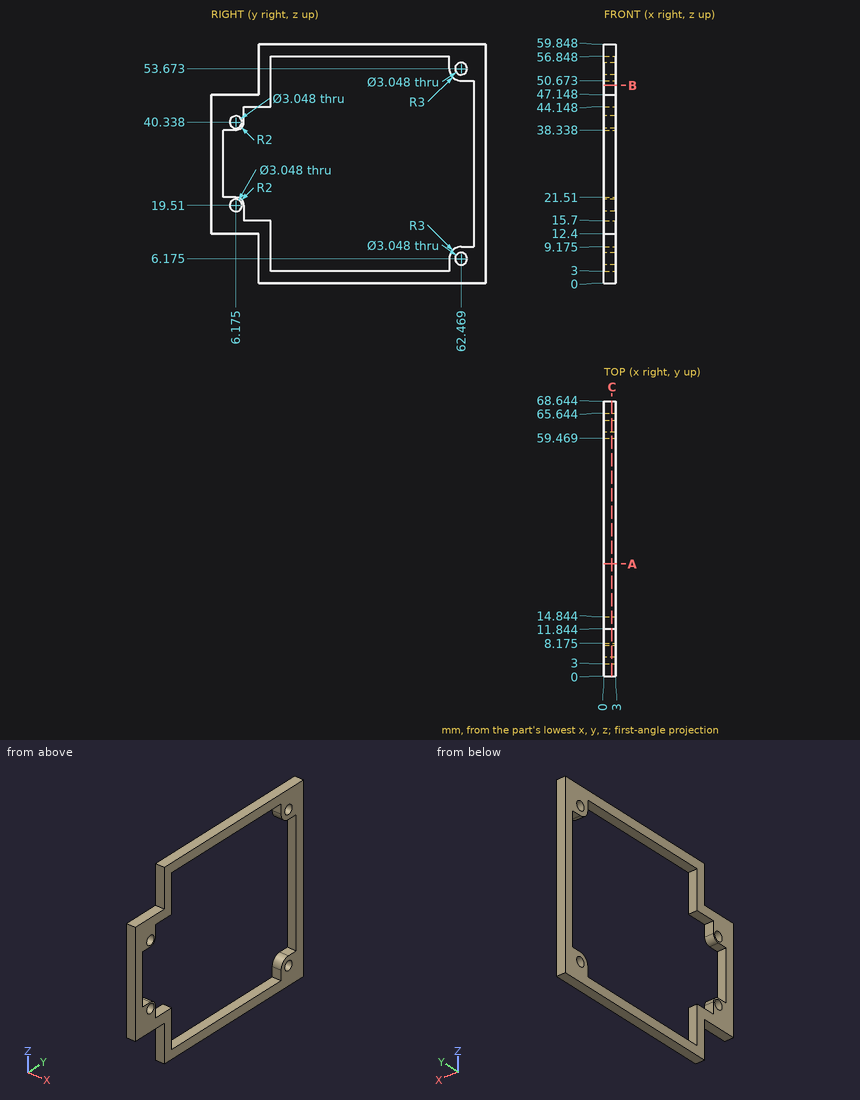
Geometry check sheet. Reference: drawing and pictorial views, mm from the part's lowest x, y, z. Round coordinates to 2 decimals unless told otherwise and drop trailing zeros. Loops run counter-clockwise (first coordinate to the right, second up) from the corner with the lowest first, then second, coordinate; pieces in that order, holes last. Notation, with made-up numbers: (87, 12.25) - (129, 12.25) arc R21 cw to (129, 39.25) - close; hole circle Ø10 at (-31.75, 21). An arc over 180 degrees is marked (long way). Write item = value, one per line. Start each with the question number.
Q1. Section check B-B (z = 49.5). Record the boundary of the cut face in (x, y).
Q2. Depth check by flat-ended pin: P1, Ø0.9, axis at x = 1, z = 55, coming from the -Y side; P2, Ø1.5, axis at x = 1, y = 3.5, coming from the +Z side; P3, Ø2.5, axis at y = 6.175, z = 40.338, coming from the -X side. Enter the tip coordinate at first touch or a pass-through.
Q3. Thickness scan on L1, parallel to Y at x = 0.9, z = 6 (1 decimal); L2, parallel to Z at x = 2.5, y = 56; L3, parallel to Y at x = 1.35, z = 17.5 (1 decimal). Record the ranges inside material, lowest first.
Q4. Section check C-C (x = 2). Count the separate pieces of the cut face and the enclosed holes in it, plus the area to 3 significant figures.
Q5. Section check A-A (y = 28). Record the boundary of the cut face in (x, z).
Derived:
q1.outline = (0, 11.84) - (3, 11.84) - (3, 14.84) - (0, 14.84) - close; (0, 65.64) - (3, 65.64) - (3, 68.64) - (0, 68.64) - close
q2.P1 = 11.84
q2.P2 = 47.15
q2.P3 = through
q3.L1 = 11.8 to 14.8, 59.5 to 61, 64 to 68.6
q3.L2 = 0 to 3, 56.85 to 59.85
q3.L3 = 0 to 8.2, 65.6 to 68.6
q4.separate_pieces = 1
q4.enclosed_holes = 5
q4.area = 840 mm^2
q5.outline = (0, 0) - (3, 0) - (3, 3) - (0, 3) - close; (0, 56.85) - (3, 56.85) - (3, 59.85) - (0, 59.85) - close
